Work out the finished part from the listing and answer in its coordinate system (mm). Face numbers are marked on the shaded views. A direction names the side the tool comes from. Round coordinates to 2 decimals unless told otherwise and drop trailing zeros. Loops run counter-clockwise (first coordinate to the right, second up) from the corner with the lowest first, then second, coordinate; pieces in that order, holes last. Notation, with made-up numbers: M -0.75,28.25 L 48.25,28.25 A26 ccw 48.25,51.25 Z; hole C -33,78.25 d6. An arc over 180 degrees is marked long. One line per item, written item: value.
```python
from build123d import *

# Parameters (mm, degrees)
SKETCH1_R                    = 50
BOSS_EXTRUDE1_DEPTH          = 40
SKETCH2_R                    = 30.75
CUT_EXTRUDE1_DEPTH           = 20
F_10_5_10_5_DIAMETER_HOLE1_D = 10.5
CUT_EXTRUDE2_DEPTH           = 82.240384046
BOSS_EXTRUDE2_START          = -3.866679
SKETCH6_W                    = 47
SKETCH6_H                    = 40
BOSS_EXTRUDE2_DEPTH          = 3.866679
BOSS_EXTRUDE3_DEPTH          = 6.5
F_9_0_9_DIAMETER_HOLE1_D     = 9
CUT_EXTRUDE3_DEPTH           = 1
CIRPATTERN1_COUNT            = 3
CIRPATTERN1_COPY_1_DEPTH     = 6.5
CIRPATTERN1_COPY_2_DEPTH     = 6.5
CIRPATTERN1_COPY_3_D         = 9
CIRPATTERN1_COPY_4_D         = 9
CUT_EXTRUDE4_DEPTH           = 1


with BuildPart() as part:
    # Sketch1 → Boss-Extrude1 (new body)
    with BuildSketch(Plane(origin=(0, 0, 0), x_dir=(1, 0, 0), z_dir=(0, 1, 0))):
        with Locations(Location((0, 0, 0), (0, 0, 270))):
            Circle(SKETCH1_R)
    extrude(amount=BOSS_EXTRUDE1_DEPTH)

    # Sketch2 → Cut-Extrude1 (cut)
    with BuildSketch(Plane(origin=(0, 40, 0), x_dir=(1, 0, 0), z_dir=(0, 1, 0))):
        with Locations(Location((0, 0, 0), (0, 0, 270))):
            Circle(SKETCH2_R)
    extrude(amount=-CUT_EXTRUDE1_DEPTH, mode=Mode.SUBTRACT)

    # Ø10.5 (10.5) Diameter Hole1 (through all)
    with Locations(Plane(origin=(0, 20, 0), x_dir=(1, 0, 0), z_dir=(0, 1, 0))):
        with Locations((0, 0)):
            Hole(F_10_5_10_5_DIAMETER_HOLE1_D / 2)

    # Sketch5 → Cut-Extrude2 (cut, through all)
    with BuildSketch(Plane(origin=(0, 40, 0), x_dir=(1, 0, 0), z_dir=(0, 1, 0))):
        with BuildLine():
            Line((-14, 48), (14, 48))
            ThreePointArc((14, 48), (0, 50), (-14, 48))
        make_face()
    cut_extrude2 = extrude(amount=-CUT_EXTRUDE2_DEPTH, mode=Mode.SUBTRACT)

    # Sketch6 → Boss-Extrude2 (add)
    with BuildSketch(Plane(origin=(0, 0, -48), x_dir=(-1, 0, 0), z_dir=(0, 0, -1)).offset(BOSS_EXTRUDE2_START)):
        with Locations((0, 20)):
            Rectangle(SKETCH6_W, SKETCH6_H)
    boss_extrude2 = extrude(amount=BOSS_EXTRUDE2_DEPTH)

    # Sketch7 → Boss-Extrude3 (add)
    with BuildSketch(Plane.ZY.offset(23.5)):
        with BuildLine():
            Line((-59, 40), (-48, 40))
            Line((-48, 40), (-48, 0))
            Line((-48, 0), (-59, 0))
            ThreePointArc((-59, 0), (-79, 20), (-59, 40))
        make_face()
    boss_extrude3 = extrude(amount=-BOSS_EXTRUDE3_DEPTH)

    # Ø9.0 (9) Diameter Hole1 (through all)
    with Locations(Plane.ZY.offset(23.5)):
        with Locations((-59, 20)):
            f_9_0_9_diameter_hole1 = Hole(F_9_0_9_DIAMETER_HOLE1_D / 2)

    # Mirror1: Boss-Extrude3, Ø9.0 (9) Diameter Hole1 across plane
    add(boss_extrude3.mirror(Plane(origin=(0, 0, 0), x_dir=(0, 0, 1), z_dir=(1, 0, 0))))
    add(f_9_0_9_diameter_hole1.mirror(Plane(origin=(0, 0, 0), x_dir=(0, 0, 1), z_dir=(1, 0, 0))), mode=Mode.SUBTRACT)

    # Sketch10 → Cut-Extrude3 (cut)
    with BuildSketch(Plane.ZY.offset(23.5)):
        with BuildLine():
            Line((-65.5, 22), (-65.5, 0))
            Line((-65.5, 0), (-52.5, 0))
            Line((-52.5, 0), (-52.5, 22))
            ThreePointArc((-52.5, 22), (-59, 28.5), (-65.5, 22))
        make_face()
    cut_extrude3 = extrude(amount=-CUT_EXTRUDE3_DEPTH, mode=Mode.SUBTRACT)

    # CirPattern1: Cut-Extrude2, Boss-Extrude2, Boss-Extrude3, Ø9.0 (9) Diameter Hole1, Cut-Extrude3 ×3 about axis
    cirpattern1_axis = Axis((0, 0, 0), (0, 1, 0))
    add([cut_extrude2.rotate(cirpattern1_axis, i * 360 / CIRPATTERN1_COUNT) for i in range(1, CIRPATTERN1_COUNT)], mode=Mode.SUBTRACT)
    add([boss_extrude2.rotate(cirpattern1_axis, i * 360 / CIRPATTERN1_COUNT) for i in range(1, CIRPATTERN1_COUNT)])
    add([boss_extrude3.rotate(cirpattern1_axis, i * 360 / CIRPATTERN1_COUNT) for i in range(1, CIRPATTERN1_COUNT)])
    add([f_9_0_9_diameter_hole1.rotate(cirpattern1_axis, i * 360 / CIRPATTERN1_COUNT) for i in range(1, CIRPATTERN1_COUNT)], mode=Mode.SUBTRACT)
    add([cut_extrude3.rotate(cirpattern1_axis, i * 360 / CIRPATTERN1_COUNT) for i in range(1, CIRPATTERN1_COUNT)], mode=Mode.SUBTRACT)

    # CirPattern1 copy 1 sketch → CirPattern1 copy 1 (add)
    with BuildSketch(Plane(origin=(-11.75, 0, -20.351596989), x_dir=(0.8660254037844387, 0, -0.4999999999999998), z_dir=(-0.4999999999999998, 0, -0.8660254037844387))):
        with BuildLine():
            Line((-59, -40), (-48, -40))
            Line((-48, -40), (-48, 0))
            Line((-48, 0), (-59, 0))
            ThreePointArc((-59, 0), (-79, -20), (-59, -40))
        make_face()
    extrude(amount=-CIRPATTERN1_COPY_1_DEPTH)

    # CirPattern1 copy 2 sketch → CirPattern1 copy 2 (add)
    with BuildSketch(Plane(origin=(-11.75, 0, 20.351596989), x_dir=(-0.8660254037844384, 0, -0.5000000000000004), z_dir=(-0.5000000000000004, 0, 0.8660254037844384))):
        with BuildLine():
            Line((-59, -40), (-48, -40))
            Line((-48, -40), (-48, 0))
            Line((-48, 0), (-59, 0))
            ThreePointArc((-59, 0), (-79, -20), (-59, -40))
        make_face()
    extrude(amount=-CIRPATTERN1_COPY_2_DEPTH)

    # CirPattern1 copy 3 (through all)
    with Locations(Plane(origin=(-11.75, 0, -20.351596989), x_dir=(0.8660254037844387, 0, -0.4999999999999998), z_dir=(-0.4999999999999998, 0, -0.8660254037844387))):
        with Locations((-59, -20)):
            Hole(CIRPATTERN1_COPY_3_D / 2)

    # CirPattern1 copy 4 (through all)
    with Locations(Plane(origin=(-11.75, 0, 20.351596989), x_dir=(-0.8660254037844384, 0, -0.5000000000000004), z_dir=(-0.5000000000000004, 0, 0.8660254037844384))):
        with Locations((-59, -20)):
            Hole(CIRPATTERN1_COPY_4_D / 2)

    # Sketch11 → Cut-Extrude4 (cut)
    with BuildSketch(Plane(origin=(0, 40, 0), x_dir=(1, 0, 0), z_dir=(0, 1, 0))):
        Polygon((-3.846153846, 35), (-3.846153846, 45), (-2.355769231, 45), (2.435897436, 37.538060897), (2.435897436, 45), (3.846153846, 45), (3.846153846, 35), (2.355769231, 35), (-2.435897436, 42.461939103), (-2.435897436, 35), align=None)
    extrude(amount=-CUT_EXTRUDE4_DEPTH, mode=Mode.SUBTRACT)


solid = part.part
```
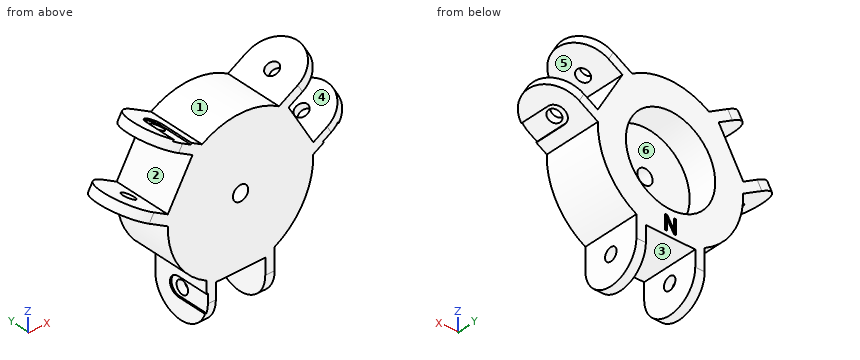
1) Find section A-A (y = 34). Give the vertices of the cut face in (x, z).
Check values:
outline: M -75.21,16.29 L -49.97,1.72 A50 ccw -23.5,-44.13 L -23.5,-73.28 L -17,-73.28 L -17,-48 L 17,-48 L 17,-73.28 L 23.5,-73.28 L 23.5,-44.13 A50 ccw 49.97,1.72 L 75.21,16.29 L 71.96,21.92 L 50.07,9.28 L 33.07,38.72 L 54.96,51.36 L 51.71,56.99 L 26.47,42.42 A50 ccw -26.47,42.42 L -51.71,56.99 L -54.96,51.36 L -33.07,38.72 L -50.07,9.28 L -71.96,21.92 Z; hole C 0,0 d61.5
2) The mould has two halves that part along Z. Classify the marked faces 1, 2 and 3: +Z half, -Z half, draft (parallel to the pull), parting line (faces both ways), or undercut.
Check values:
face 1: +Z half
face 2: undercut
face 3: -Z half
3) Find section C-C (z = -40). Give the vertices of the cut face in (x, y), then the cut area to 3 significant figures.
Check values:
outline: M -30,0 L 30,0 L 30,40 L 3.85,40 L 3.85,39 L 2.44,39 L 2.44,40 L 0.85,40 L 0.85,39 L -0.85,39 L -0.85,40 L -2.44,40 L -2.44,39 L -3.85,39 L -3.85,40 L -30,40 Z
area: 2,400 mm2
4) For the marked faces 4, 5 and 6, determine the directions among +Z, -Z, +X, -X, +Y, -Y from which every point of the face is accessible in a straight line to the end or side of a thin tool.
Check values:
face 4: +Y, -Y
face 5: +X, +Y, -Y
face 6: +Y
5) Find section B-B (x = 0). Give the vertices of the cut face in (y, z).
Check values:
outline: M 0,-48 L 40,-48 L 40,-41.33 L 39,-41.33 L 39,-38.67 L 40,-38.67 L 40,-30.75 L 20,-30.75 L 20,-5.25 L 0,-5.25 Z; M 0,5.25 L 20,5.25 L 20,30.75 L 40,30.75 L 40,50 L 0,50 Z
6) Each of these flat-tipped pins is pushed along its axis until it touches: pin 1 (0.8 mm diameter, centred on x = -23, y = 8.5, fed in from -Z); pin 2 (4 mm diameter, centred on y = 16.5, z = -57.5, fed in from -X); pin 3 (0.5 mm diameter, centred on y = 39.5, z = -41.5, fed in from -X); pin 4 (9.5 mm diameter, centred on x = 0, z = 0, fed in from +Y). Where does it stop, or does it pass through?
Check values:
pin 1: z = -75.64
pin 2: x = -22.5
pin 3: x = -28.26
pin 4: through
7) Find the intervals of material crossed by probe 1 along X at (y, z) = (36, -62.5); probe 2 along Y at (x, z) = (-20.6, -59); probe 3 along Z at (x, y) = (0, 15), in increasing order. Write a range as from..to.
Check values:
probe 1: -23.5..-17, 17..23.5
probe 2: 0..15.5, 24.5..40
probe 3: -48..-5.25, 5.25..50
